Source: CAD feature listing. Evaluate the final solid. Frame: model axes, mm. A direction names the side the tool comes from. Round coordinates to 2 decimals unless told otherwise and drop trailing zeros. Write each loop counter-clockwise with the first axis right and the second up, starting at its lowest first coordinate (ties: lowest second). Pieces come first, ordered by that corner, then holes. Notation, with made-up numbers: (-33, 59) -> (-13, 59) arc R4 cw to (-13, 64) -> close; hole circle Ø11 at (-20, 9). An arc over 180 degrees is marked (long way). Return JSON: item names as keys, results as strings. Group by question number.
from build123d import *

# Parameters (mm, degrees)
BOSS_EXTRUDE1_DEPTH      = 5
BOSS_EXTRUDE3_DEPTH      = 22.5
CUT_EXTRUDE3_DEPTH       = 21.5
CUT_EXTRUDE3_DEPTH_BACK  = 4
SKETCH2_W                = 100
SKETCH2_H                = 5
BOSS_EXTRUDE2_DEPTH      = 50
SKETCH4_R                = 5
CUT_EXTRUDE1_DEPTH       = 8.5
SKETCH5_W                = 41.64031781
SKETCH5_H                = 1
CUT_EXTRUDE2_DEPTH       = 4
BOSS_EXTRUDE5_DEPTH      = 5
BOSS_EXTRUDE5_DEPTH_BACK = 5
BOSS_EXTRUDE6_DEPTH      = 5
BOSS_EXTRUDE6_DEPTH_BACK = 5


with BuildPart() as part:
    # Sketch1 → Boss-Extrude1 (new body)
    with BuildSketch(Plane.XY):
        Polygon((25, 130), (-25, 130), (-50, 0), (-50, -5), (50, -5), (50, 0), align=None)
    extrude(amount=BOSS_EXTRUDE1_DEPTH)

    # Sketch3 → Boss-Extrude3 (add)
    with BuildSketch(Plane.XY.offset(5)):
        with BuildLine():
            Line((-15, 120), (15, 120))
            ThreePointArc((15, 120), (0, 105), (-15, 120))
        make_face()
    extrude(amount=BOSS_EXTRUDE3_DEPTH)

    # Sketch12 → Cut-Extrude3 (cut, two sides)
    with BuildSketch(Plane.XY.offset(5)) as cut_extrude3_sk:
        with BuildLine():
            Line((-14, 120), (-14, 130))
            Line((-14, 130), (14, 130))
            Line((14, 130), (14, 120))
            ThreePointArc((14, 120), (0, 106), (-14, 120))
        make_face()
    extrude(amount=CUT_EXTRUDE3_DEPTH, mode=Mode.SUBTRACT)
    extrude(cut_extrude3_sk.sketch, amount=-CUT_EXTRUDE3_DEPTH_BACK, mode=Mode.SUBTRACT)

    # Sketch2 → Boss-Extrude2 (add)
    with BuildSketch(Plane.XY.offset(5)):
        with Locations((0, -2.5)):
            Rectangle(SKETCH2_W, SKETCH2_H)
    extrude(amount=BOSS_EXTRUDE2_DEPTH)

    # Sketch4 → Cut-Extrude1 (cut)
    with BuildSketch(Plane.XY.offset(27.5)):
        with Locations((0, 111)):
            Circle(SKETCH4_R)
    extrude(amount=-CUT_EXTRUDE1_DEPTH, mode=Mode.SUBTRACT)

    # Sketch5 → Cut-Extrude2 (cut)
    with BuildSketch(Plane(origin=(0, 120, 0), x_dir=(1, 0, 0), z_dir=(0, 1, 0))):
        with Locations((0.627254623, -25.5)):
            Rectangle(SKETCH5_W, SKETCH5_H)
    extrude(amount=-CUT_EXTRUDE2_DEPTH, mode=Mode.SUBTRACT)

    # Sketch8 → Boss-Extrude5 (add, two sides)
    with BuildSketch(Plane(origin=(-35, 0, 0), x_dir=(0, 0, -1), z_dir=(1, 0, 0))) as boss_extrude5_sk:
        with BuildLine():
            Line((-40.75, 3.25), (-40.75, 0))
            Line((-40.75, 0), (-55, 0))
            Line((-55, 0), (-55, -5))
            Line((-55, -5), (0, -5))
            Line((0, -5), (0, 0))
            Line((0, 0), (-5, 0))
            Line((-5, 0), (-32.25, 0))
            Line((-32.25, 0), (-32.25, 3.25))
            Line((-32.25, 3.25), (-33.616859351, 4.75))
            ThreePointArc((-33.616859351, 4.75), (-36.5, 0), (-39.383140649, 4.75))
            Line((-39.383140649, 4.75), (-40.75, 3.25))
        make_face()
    extrude(amount=BOSS_EXTRUDE5_DEPTH)
    extrude(boss_extrude5_sk.sketch, amount=-BOSS_EXTRUDE5_DEPTH_BACK)

    # Sketch11 → Boss-Extrude6 (add, two sides)
    with BuildSketch(Plane(origin=(35, 0, 0), x_dir=(0, 0, -1), z_dir=(1, 0, 0))) as boss_extrude6_sk:
        with BuildLine():
            Line((-40.75, 3.25), (-40.75, 0))
            Line((-40.75, 0), (-55, 0))
            Line((-55, 0), (-55, -5))
            Line((-55, -5), (0, -5))
            Line((0, -5), (0, 0))
            Line((0, 0), (-5, 0))
            Line((-5, 0), (-32.25, 0))
            Line((-32.25, 0), (-32.25, 3.25))
            Line((-32.25, 3.25), (-33.616859351, 4.75))
            ThreePointArc((-33.616859351, 4.75), (-36.5, 0), (-39.383140649, 4.75))
            Line((-39.383140649, 4.75), (-40.75, 3.25))
        make_face()
    extrude(amount=BOSS_EXTRUDE6_DEPTH)
    extrude(boss_extrude6_sk.sketch, amount=-BOSS_EXTRUDE6_DEPTH_BACK)


solid = part.part
Item 1: Cut plane B-B on x = 37.5. Output: boundary loops of the cut face in (y, z).
Item 2: Pull-direction query (Z, two-part tool) for faces 1 (the flat face through (1, -2, 55)), 2 (the flat face through (-37.325, 65.91, 2.465)), 3 (the flat face through (35, 2, 32.25)); classes: +Z half, -Z half, draft (parallel to the pull), parting line (faces both ways), or undercut.
Item 3: Set-up query: faces 4 (the cylindrical face through (0, 106, 14)), 5 (the flat face through (-40, 2, 33)), 6 (the flat face through (-14, 125, 3)), 7 (the flat face through (40, 2, 33)). Return all of +Z, -Z, +X, -X, +Y, -Y with unobstructed straight access to the full face (end or side cutting, diameter ignored); none if empty.
Item 4: Cut plane A-A on x = 3. Output: boundary loops of the cut face in (y, z), and give its area (3 significant figures).
Item 5: Cut plane D-D on z = 47. Output: boundary loops of the cut face in (x, y), and give its area (3 significant figures).
Item 6: Material intervals for probe 1 along Z at (x, y) = (-34.75, 3.25); probe 2 along Y at (x, z) = (0, 27); probe 3 along Z at (x, y) = (32, 3), sorted ascending.
Item 7: Cut plane C-C on y = 111. Output: boundary loops of the cut face in (x, z), and give its area (3 significant figures).
Item 8: First-contact query: pin 1 Ø4 at (x, z) = (-38.5, 43) entering from +Y; pin 2 Ø15.5 at (x, y) = (5.5, 112) entering from -Z; pin 3 Ø3 at (x, z) = (5.5, 12) entering from +Y; pin 4 Ø1.2 at (y, z) = (124.5, 3) entering from +X. Flat tips, straight axial feed; report the tip coordinate or a pass-through.
Here are the results:
{
 "1": {"outline": "(-5, 0) -> (65, 0) -> (65, 5) -> (0, 5) -> (0, 32.25) -> (3.25, 32.25) -> (4.75, 33.62) arc R3.25 cw (long way) to (4.75, 39.38) -> (3.25, 40.75) -> (0, 40.75) -> (0, 55) -> (-5, 55) -> close"},
 "2": {"face 1": "+Z half", "face 2": "draft", "face 3": "undercut"},
 "3": {"face 4": "+Y", "face 5": "+Z, -X, +Y", "face 6": "+Z, +Y", "face 7": "+Z, +X, +Y"},
 "4": {"outline": "(-5, 0) -> (130, 0) -> (130, 1) -> (106.33, 1) -> (106.33, 26.5) -> (107, 26.5) -> (107, 27.5) -> (105.3, 27.5) -> (105.3, 5) -> (0, 5) -> (0, 55) -> (-5, 55) -> close; (115, 26.5) -> (120, 26.5) -> (120, 27.5) -> (115, 27.5) -> close", "area": "859 mm^2"},
 "5": {"outline": "(-50, -5) -> (50, -5) -> (50, 0) -> (-50, 0) -> close", "area": "500 mm^2"},
 "6": {"probe 1": "z = 0 to 5, 32.25 to 33.25, 39.75 to 40.75", "probe 2": "y = -5 to 0, 105 to 106, 116 to 120", "probe 3": "z = 0 to 5, 32.25 to 33.26, 39.74 to 40.75"},
 "7": {"outline": "(-28.65, 0) -> (28.65, 0) -> (28.65, 5) -> (12, 5) -> (12, 27.5) -> (5, 27.5) -> (5, 26.5) -> (10.72, 26.5) -> (10.72, 1) -> (-10.72, 1) -> (-10.72, 26.5) -> (-5, 26.5) -> (-5, 27.5) -> (-12, 27.5) -> (-12, 5) -> (-28.65, 5) -> close", "area": "270 mm^2"},
 "8": {"pin 1": "stops at y = 0", "pin 2": "stops at z = 0", "pin 3": "stops at y = 107.88", "pin 4": "stops at x = 26.17"}
}
